Job drawing, mm, ordinate dimensions from the low corner. One solid piece. A direction names the side the tool comes from. Give positions to 0.01 mm unless a question says otherwise; leave off trailing zeros. Order: outer loops, then holes, each group sorted by start corner. A loop starts at its lowest first (then second) coordinate and runs counter-clockwise, first axis right, second up.
1. Which spindle directions (+Z, -Z, +X, -X, +Y, -Y) get a long thin tool onto all of the face, cutting with end or side? Do the marked faces 1, 2, 3 and 4. Say none if no direction does.
2. Slice it at B-B on z = 20. List the corners of the cut face in (x, y), and give its area (3 significant figures).
3. Slice it at D-D on x = 10. List the corners of the cut face in (y, z).
4. Probe line 1 (X direction, y = 18, z = 22); line 2 (Y direction, x = 3, z = 19.5). List the from-to ranges inside material, lowest first.
5. Drop flat-ended pins along their axis: pin 1 Ø6 at (x, z) = (52.5, 18) entering from +Y; pin 2 Ø1.5 at (x, y) = (9, 33) entering from -Z; pin 3 Ø4 at (y, z) = (26.5, 33) entering from +X. Give the stop position or say it passes through.
6. Slice it at A-A on x = 37.5. List the corners of the cut face in (y, z), and give its area (4 significant figures).
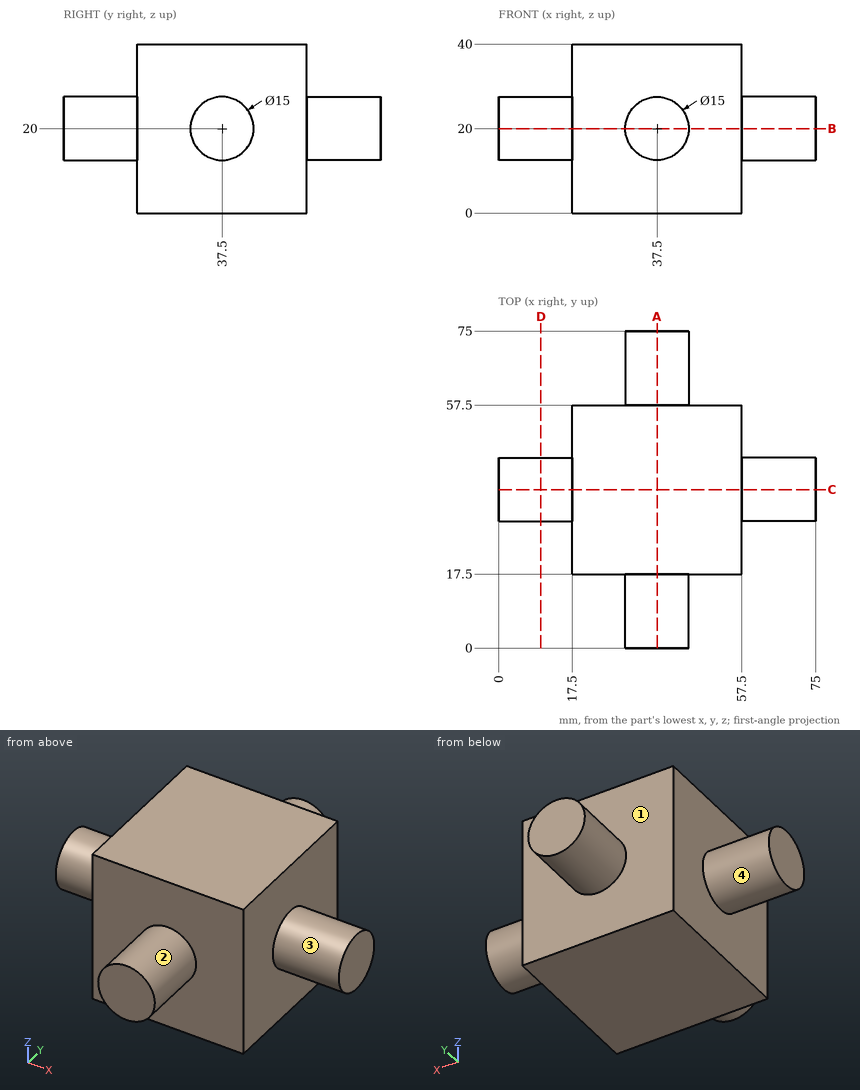
Data:
1. face 1: +Y
1. face 2: -Y
1. face 3: +X
1. face 4: -X
2. outline: (0, 30) - (17.5, 30) - (17.5, 17.5) - (30, 17.5) - (30, 0) - (45, 0) - (45, 17.5) - (57.5, 17.5) - (57.5, 30) - (75, 30) - (75, 45) - (57.5, 45) - (57.5, 57.5) - (45, 57.5) - (45, 75) - (30, 75) - (30, 57.5) - (17.5, 57.5) - (17.5, 45) - (0, 45) - close
2. area: 2,650 mm2
3. outline: circle Ø15 at (37.5, 20)
4. line 1: x = 17.5 to 57.5
4. line 2: y = 30.02 to 44.98
5. pin 1: stops at y = 57.5
5. pin 2: stops at z = 13.5
5. pin 3: stops at x = 57.5
6. outline: (0, 12.5) - (17.5, 12.5) - (17.5, 0) - (57.5, 0) - (57.5, 12.5) - (75, 12.5) - (75, 27.5) - (57.5, 27.5) - (57.5, 40) - (17.5, 40) - (17.5, 27.5) - (0, 27.5) - close
6. area: 2,125 mm2
